Input: part model. Units: mm. Frame: model coordinates. Coordinates: 2 decimals unless noted, no trailing zeros. Write each loop counter-clockwise with the first axis right and the second up, starting at its lowest first coordinate (ties: lowest second). Pieces come first, ordered by that corner, then holes. Notation, with made-up numbers: M 15.5,-3.5 L 21.5,-3.5 A14 ccw 21.5,6.5 Z; hole C -32.5,10.25 d9. An arc over 180 degrees is marked long. Use CSV: the item, a comma, the result in double quotes.
```python
from build123d import *

# Parameters (mm, degrees)
F0_R     = 45.72
F1_DEPTH = 76.2
F2_DEPTH = 12.7


with BuildPart() as f1:
    # F0 (on Front) → F1 (new body, symmetric)
    with BuildSketch(Plane.XZ):
        Circle(F0_R)
        with BuildLine():
            ThreePointArc((44.4318571429, 1.2698704016), (44.4454640543, 0.635), (44.45, 0))
            ThreePointArc((44.45, 0), (44.4454640543, -0.635), (44.4318571429, -1.2698704016))
            ThreePointArc((44.4318571429, -1.2698704016), (31.4308964237, -31.4308964237), (1.2698704016, -44.4318571429))
            ThreePointArc((1.2698704016, -44.4318571429), (0.635, -44.4454640543), (0, -44.45))
            ThreePointArc((0, -44.45), (-0.635, -44.4454640543), (-1.2698704016, -44.4318571429))
            ThreePointArc((-1.2698704016, -44.4318571429), (-31.4308964237, -31.4308964237), (-44.4318571429, -1.2698704016))
            ThreePointArc((-44.4318571429, -1.2698704016), (-44.4454640543, -0.635), (-44.45, 0))
            ThreePointArc((-44.45, 0), (-44.4454640543, 0.635), (-44.4318571429, 1.2698704016))
            ThreePointArc((-44.4318571429, 1.2698704016), (-31.4308964237, 31.4308964237), (-1.2698704016, 44.4318571429))
            ThreePointArc((-1.2698704016, 44.4318571429), (-0.635, 44.4454640543), (0, 44.45))
            ThreePointArc((0, 44.45), (0.635, 44.4454640543), (1.2698704016, 44.4318571429))
            ThreePointArc((1.2698704016, 44.4318571429), (31.4308964237, 31.4308964237), (44.4318571429, 1.2698704016))
        make_face(mode=Mode.SUBTRACT)
    extrude(amount=F1_DEPTH, both=True)

    # F0 (on Front) → F2 (join, symmetric)
    with BuildSketch(Plane.XZ):
        with BuildLine():
            Line((-12.6363534757, 1.2698704016), (-13.7860050542, 1.2698704016))
            ThreePointArc((-13.7860050542, 1.2698704016), (-13.8297690489, 0.635605418), (-13.8443673092, 0))
            Line((-13.8443673092, 0), (-12.7, 0))
            ThreePointArc((-12.7, 0), (-12.6840783887, 0.6357321993), (-12.6363534757, 1.2698704016))
        make_face()
        with BuildLine():
            Line((-13.7860050542, 1.2698704016), (-44.4318571429, 1.2698704016))
            ThreePointArc((-44.4318571429, 1.2698704016), (-44.4454640543, 0.635), (-44.45, 0))
            Line((-44.45, 0), (-13.8443673092, 0))
            ThreePointArc((-13.8443673092, 0), (-13.8297690489, 0.635605418), (-13.7860050542, 1.2698704016))
        make_face()
        with BuildLine():
            Line((1.2698704016, 12.6363534757), (1.2698704016, 13.7860050542))
            ThreePointArc((1.2698704016, 13.7860050542), (0.635605418, 13.8297690489), (0, 13.8443673092))
            Line((0, 13.8443673092), (0, 12.7))
            ThreePointArc((0, 12.7), (0.6357321993, 12.6840783887), (1.2698704016, 12.6363534757))
        make_face()
        with BuildLine():
            Line((1.2698704016, 13.7860050542), (1.2698704016, 44.4318571429))
            ThreePointArc((1.2698704016, 44.4318571429), (0.635, 44.4454640543), (0, 44.45))
            Line((0, 44.45), (0, 13.8443673092))
            ThreePointArc((0, 13.8443673092), (0.635605418, 13.8297690489), (1.2698704016, 13.7860050542))
        make_face()
        with BuildLine():
            Line((12.7, 0), (13.8443673092, 0))
            ThreePointArc((13.8443673092, 0), (13.8297690489, 0.635605418), (13.7860050542, 1.2698704016))
            Line((13.7860050542, 1.2698704016), (12.6363534757, 1.2698704016))
            ThreePointArc((12.6363534757, 1.2698704016), (12.6840783887, 0.6357321993), (12.7, 0))
        make_face()
        with BuildLine():
            Line((13.8443673092, 0), (44.45, 0))
            ThreePointArc((44.45, 0), (44.4454640543, 0.635), (44.4318571429, 1.2698704016))
            Line((44.4318571429, 1.2698704016), (13.7860050542, 1.2698704016))
            ThreePointArc((13.7860050542, 1.2698704016), (13.8297690489, 0.635605418), (13.8443673092, 0))
        make_face()
        with BuildLine():
            ThreePointArc((-1.2698704016, -13.7860050542), (-0.635605418, -13.8297690489), (0, -13.8443673092))
            Line((0, -13.8443673092), (0, -12.7))
            ThreePointArc((0, -12.7), (-0.6357321993, -12.6840783887), (-1.2698704016, -12.6363534757))
            Line((-1.2698704016, -12.6363534757), (-1.2698704016, -13.7860050542))
        make_face()
        with BuildLine():
            ThreePointArc((-1.2698704016, -44.4318571429), (-0.635, -44.4454640543), (0, -44.45))
            Line((0, -44.45), (0, -13.8443673092))
            ThreePointArc((0, -13.8443673092), (-0.635605418, -13.8297690489), (-1.2698704016, -13.7860050542))
            Line((-1.2698704016, -13.7860050542), (-1.2698704016, -44.4318571429))
        make_face()
        with BuildLine():
            ThreePointArc((0, -13.8443673092), (0.635605418, -13.8297690489), (1.2698704016, -13.7860050542))
            Line((1.2698704016, -13.7860050542), (1.2698704016, -12.6363534757))
            ThreePointArc((1.2698704016, -12.6363534757), (0.6357321993, -12.6840783887), (0, -12.7))
            Line((0, -12.7), (0, -13.8443673092))
        make_face()
        with BuildLine():
            ThreePointArc((0, -44.45), (0.635, -44.4454640543), (1.2698704016, -44.4318571429))
            Line((1.2698704016, -44.4318571429), (1.2698704016, -13.7860050542))
            ThreePointArc((1.2698704016, -13.7860050542), (0.635605418, -13.8297690489), (0, -13.8443673092))
            Line((0, -13.8443673092), (0, -44.45))
        make_face()
        with BuildLine():
            ThreePointArc((-13.8443673092, 0), (-13.8297690489, -0.635605418), (-13.7860050542, -1.2698704016))
            Line((-13.7860050542, -1.2698704016), (-12.6363534757, -1.2698704016))
            ThreePointArc((-12.6363534757, -1.2698704016), (-12.6840783887, -0.6357321993), (-12.7, 0))
            Line((-12.7, 0), (-13.8443673092, 0))
        make_face()
        with BuildLine():
            ThreePointArc((-44.45, 0), (-44.4454640543, -0.635), (-44.4318571429, -1.2698704016))
            Line((-44.4318571429, -1.2698704016), (-13.7860050542, -1.2698704016))
            ThreePointArc((-13.7860050542, -1.2698704016), (-13.8297690489, -0.635605418), (-13.8443673092, 0))
            Line((-13.8443673092, 0), (-44.45, 0))
        make_face()
        with BuildLine():
            ThreePointArc((13.7860050542, -1.2698704016), (13.8297690489, -0.635605418), (13.8443673092, 0))
            Line((13.8443673092, 0), (12.7, 0))
            ThreePointArc((12.7, 0), (12.6840783887, -0.6357321993), (12.6363534757, -1.2698704016))
            Line((12.6363534757, -1.2698704016), (13.7860050542, -1.2698704016))
        make_face()
        with BuildLine():
            ThreePointArc((44.4318571429, -1.2698704016), (44.4454640543, -0.635), (44.45, 0))
            Line((44.45, 0), (13.8443673092, 0))
            ThreePointArc((13.8443673092, 0), (13.8297690489, -0.635605418), (13.7860050542, -1.2698704016))
            Line((13.7860050542, -1.2698704016), (44.4318571429, -1.2698704016))
        make_face()
        with BuildLine():
            ThreePointArc((-13.7860050542, -1.2698704016), (-9.7894460056, -9.7894460056), (-1.2698704016, -13.7860050542))
            Line((-1.2698704016, -13.7860050542), (-1.2698704016, -12.6363534757))
            ThreePointArc((-1.2698704016, -12.6363534757), (-8.9802561211, -8.9802561211), (-12.6363534757, -1.2698704016))
            Line((-12.6363534757, -1.2698704016), (-13.7860050542, -1.2698704016))
        make_face()
        with BuildLine():
            ThreePointArc((1.2698704016, -13.7860050542), (9.7894460056, -9.7894460056), (13.7860050542, -1.2698704016))
            Line((13.7860050542, -1.2698704016), (12.6363534757, -1.2698704016))
            ThreePointArc((12.6363534757, -1.2698704016), (8.9802561211, -8.9802561211), (1.2698704016, -12.6363534757))
            Line((1.2698704016, -12.6363534757), (1.2698704016, -13.7860050542))
        make_face()
        with BuildLine():
            Line((12.6363534757, 1.2698704016), (13.7860050542, 1.2698704016))
            ThreePointArc((13.7860050542, 1.2698704016), (9.7894460056, 9.7894460056), (1.2698704016, 13.7860050542))
            Line((1.2698704016, 13.7860050542), (1.2698704016, 12.6363534757))
            ThreePointArc((1.2698704016, 12.6363534757), (8.9802561211, 8.9802561211), (12.6363534757, 1.2698704016))
        make_face()
        with BuildLine():
            Line((-1.2698704016, 12.6363534757), (-1.2698704016, 13.7860050542))
            ThreePointArc((-1.2698704016, 13.7860050542), (-9.7894460056, 9.7894460056), (-13.7860050542, 1.2698704016))
            Line((-13.7860050542, 1.2698704016), (-12.6363534757, 1.2698704016))
            ThreePointArc((-12.6363534757, 1.2698704016), (-8.9802561211, 8.9802561211), (-1.2698704016, 12.6363534757))
        make_face()
        with BuildLine():
            Line((0, 13.8443673092), (0, 44.45))
            ThreePointArc((0, 44.45), (-0.635, 44.4454640543), (-1.2698704016, 44.4318571429))
            Line((-1.2698704016, 44.4318571429), (-1.2698704016, 13.7860050542))
            ThreePointArc((-1.2698704016, 13.7860050542), (-0.635605418, 13.8297690489), (0, 13.8443673092))
        make_face()
        with BuildLine():
            Line((0, 12.7), (0, 13.8443673092))
            ThreePointArc((0, 13.8443673092), (-0.635605418, 13.8297690489), (-1.2698704016, 13.7860050542))
            Line((-1.2698704016, 13.7860050542), (-1.2698704016, 12.6363534757))
            ThreePointArc((-1.2698704016, 12.6363534757), (-0.6357321993, 12.6840783887), (0, 12.7))
        make_face()
    extrude(amount=F2_DEPTH, both=True)


solid = f1.part
```
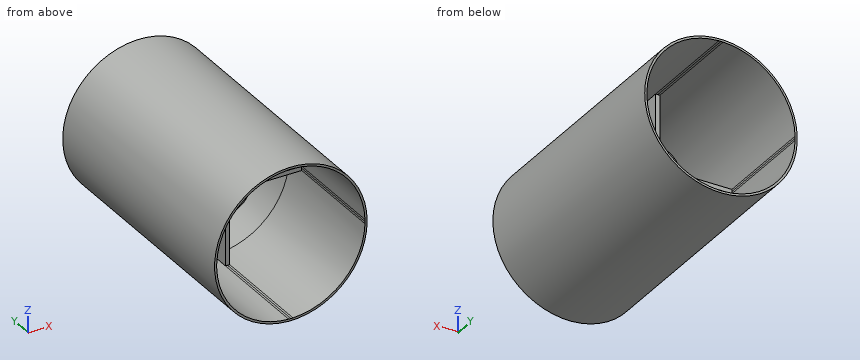
1. Section D-D (x = 38.5). Return loops of the section in (y, z).
Resolved:
outline,"M -76.2,-24.66 L 76.2,-24.66 L 76.2,-22.22 L -76.2,-22.22 Z; M -76.2,22.22 L 76.2,22.22 L 76.2,24.66 L -76.2,24.66 Z; M -12.7,-1.27 L 12.7,-1.27 L 12.7,1.27 L -12.7,1.27 Z"
2. Contact query for flat-ended pins moving along their axis: pin 1 Ø12.5 at (y, z) = (2.5, 24.5) entering from +X; pin 2 Ø2 at (x, y) = (-8.5, -2) entering from -Z; pin 3 Ø20.5 at (y, z) = (1.5, -36) entering from -X. Output: stop coordinate, or through.
Resolved:
pin 1,"stops at x = 41.92"
pin 2,"stops at z = -45.1"
pin 3,"stops at x = -37.78"
3. Section B-B (y = -3). Return loops of the section in (x, z), then the cut area to 3 significant figures.
Resolved:
outline,"C 0,0 d91.44; hole M -44.43,-1.27 A44.45 ccw -1.27,-44.43 L -1.27,-13.79 A13.84 cw -13.79,-1.27 Z; hole M -44.43,1.27 L -13.79,1.27 A13.84 cw -1.27,13.79 L -1.27,44.43 A44.45 ccw Z; hole C 0,0 d25.4; hole M 1.27,-44.43 A44.45 ccw 44.43,-1.27 L 13.79,-1.27 A13.84 cw 1.27,-13.79 Z; hole M 1.27,13.79 A13.84 cw 13.79,1.27 L 44.43,1.27 A44.45 ccw 1.27,44.43 Z"
area,"766 mm^2"
4. Material intervals for line 1 (Z direction, x = 0.5, y = -18); line 2 (X direction, y = 1.5, z = -14); line 3 (Z direction, x = 36.5, y = 2), sorted ascending. Write a range as [from, to].
Resolved:
line 1,"z = [-45.72, -44.45], [44.45, 45.72]"
line 2,"x = [-43.52, -42.19], [-1.27, 1.27], [42.19, 43.52]"
line 3,"z = [-27.53, -25.37], [-1.27, 1.27], [25.37, 27.53]"
5. Section A-A (y = 39). Return loops of the section in (x, z), then the cut area to 3 significant figures.
Resolved:
outline,"C 0,0 d91.44; hole C 0,0 d88.9"
area,"360 mm^2"
6. Section C-C (z = 20). Return loops of the section in (x, y).
Resolved:
outline,"M -41.11,-76.2 L -39.7,-76.2 L -39.7,76.2 L -41.11,76.2 Z; M -1.27,-12.7 L 1.27,-12.7 L 1.27,12.7 L -1.27,12.7 Z; M 39.7,-76.2 L 41.11,-76.2 L 41.11,76.2 L 39.7,76.2 Z"
